```python
from build123d import *

# Parameters (mm, degrees)
F0_W     = 150
F0_H     = 150
F1_DEPTH = 3
F2_D     = 6.7564
F4_DEPTH = 25


with BuildPart() as f1:
    # F0 (on Top) → F1 (new body)
    with BuildSketch(Plane.XY):
        with Locations((0, 1.9158130744)):
            Rectangle(F0_W, F0_H)
    extrude(amount=F1_DEPTH)

    # F2 (through all)
    with Locations(Plane(origin=(0, 0, 0), x_dir=(1, 0, 0), z_dir=(0, 0, -1))):
        with Locations((-26.6683554199, -56.9034204527), (26.6683554199, -56.9034204527), (-26.6683554199, 6.102117215), (26.6683554199, 6.102117215)):
            Hole(F2_D / 2)

    # F3 (on face) → F4 (cut)
    with BuildSketch(Plane.XY.offset(3)):
        with BuildLine():
            Line((-3.7946185299, 58.3347232517), (-30.747280214, 37.7231456992))
            ThreePointArc((-30.747280214, 37.7231456992), (-32.2234435202, 33.0477107055), (-32.9929459562, 28.2055400674))
            Line((-32.9929459562, 28.2055400674), (5.9788893458, 58.0085708442))
            ThreePointArc((5.9788893458, 58.0085708442), (1.1042434503, 58.5344775669), (-3.7946185299, 58.3347232517))
        make_face()
        with BuildLine():
            Line((13.2642979666, 55.7796879625), (-32.7505124435, 20.5906649099))
            ThreePointArc((-32.7505124435, 20.5906649099), (-32.0865867054, 17.2832595371), (-31.0895548602, 14.0605812744))
            Line((-31.0895548602, 14.0605812744), (19.1311825167, 52.4660135586))
            ThreePointArc((19.1311825167, 52.4660135586), (16.2822571669, 54.2724885893), (13.2642979666, 55.7796879625))
        make_face()
        with BuildLine():
            Line((23.9241830701, 48.3311051134), (-28.3547132801, 8.3517316803))
            ThreePointArc((-28.3547132801, 8.3517316803), (-26.6305999484, 5.7731261787), (-24.6727303472, 3.3671919031))
            Line((-24.6727303472, 3.3671919031), (27.7700422707, 43.4718868513))
            ThreePointArc((27.7700422707, 43.4718868513), (25.96105225, 45.9916741873), (23.9241830701, 48.3311051134))
        make_face()
        with BuildLine():
            Line((30.6779404767, 37.8953792911), (-20.0527864197, -0.900058576))
            ThreePointArc((-20.0527864197, -0.900058576), (-17.3098813008, -2.7781418823), (-14.3924694915, -4.371701963))
            Line((-14.3924694915, -4.371701963), (32.545465682, 31.5232646388))
            ThreePointArc((32.545465682, 31.5232646388), (31.7718544133, 34.7562587621), (30.6779404767, 37.8953792911))
        make_face()
        with BuildLine():
            Line((33.0822923496, 24.1335215078), (-7.4014540257, -6.8257168713))
            ThreePointArc((-7.4014540257, -6.8257168713), (-2.8461445024, -7.5410678745), (1.7643727579, -7.6165827867))
            Line((1.7643727579, -7.6165827867), (31.4443076996, 15.0806293838))
            ThreePointArc((31.4443076996, 15.0806293838), (32.5792762723, 19.5499042969), (33.0822923496, 24.1335215078))
        make_face()
    extrude(amount=-F4_DEPTH, mode=Mode.SUBTRACT)


solid = f1.part
```
Input: part model. Units: mm. Frame: model coordinates. A direction names the side the tool comes from. Give positions to 0.01 mm unless a question says otherwise; leave off trailing zeros. Order: outer loops, then holes, each group sorted by start corner. A loop starts at its lowest first (then second) coordinate and runs counter-clockwise, first axis right, second up. Notation, with made-up numbers: M 36,49 L 59,49 A20 ccw 59,86 Z; hole C -15,-30 d10. An arc over 180 degrees is marked long. Return JSON: item names as keys, results as strings.
Item 1: Access query for faces 1 (the flat face through (-1, 3, 3)), 2 (the flat face through (-9.42, 38.43, 1.52)). Directions: +Z, -Z, +X, -X, +Y, -Y. A direction counts if a zero-diameter tool reaches every point of the face in a straight line with its end or side. Return the directions, or none.
Solutions:
{"face 1": "+Z, +X, -X, +Y, -Y", "face 2": "+Z, -Z"}
Item 2: Cut plane A-A (x = -1.5). Return loops of the section in (y, z), then the cut area to 3 significant figures.
Solutions:
{"outline": "M -73.08,0 L -7.63,0 L -7.63,3 L -73.08,3 Z; M -2.31,0 L 5.49,0 L 5.49,3 L -2.31,3 Z; M 13.29,0 L 21.09,0 L 21.09,3 L 13.29,3 Z; M 28.89,0 L 36.69,0 L 36.69,3 L 28.89,3 Z; M 44.49,0 L 52.29,0 L 52.29,3 L 44.49,3 Z; M 58.52,0 L 76.92,0 L 76.92,3 L 58.52,3 Z", "area": "345 mm^2"}
Item 3: Ray query, probe 1 along X at (y, z) = (-2, 2.05); probe 2 along X at (y, z) = (-9, 2.9); probe 3 along X at (y, z) = (10.5, 2.2). Return the intervals inside material, ascending.
Solutions:
{"probe 1": "-75 to -18.52, -11.29 to -1.09, 9.11 to 75", "probe 2": "-75 to -28.4, -24.93 to 24.93, 28.4 to 75", "probe 3": "-75 to -25.55, -15.35 to -5.15, 5.05 to 15.25, 25.45 to 75"}
Item 4: Pull-direction query (Y, two-part tool) for faces 3 (the flat face through (-1, 3, 0)), 4 (the flat face through (16.397, 3.573, 1.521)); classes: +Y half, -Y half, draft (parallel to the pull), parting line (faces both ways), or undercut.
Solutions:
{"face 3": "draft", "face 4": "undercut"}
Item 5: Cut plane B-B (z = 1.5). State how many separate pieces and enclosed holes the cut face has, then the cut area to 3 significant figures.
Solutions:
{"separate pieces": "1", "enclosed holes": "9", "area": "20,600 mm^2"}
